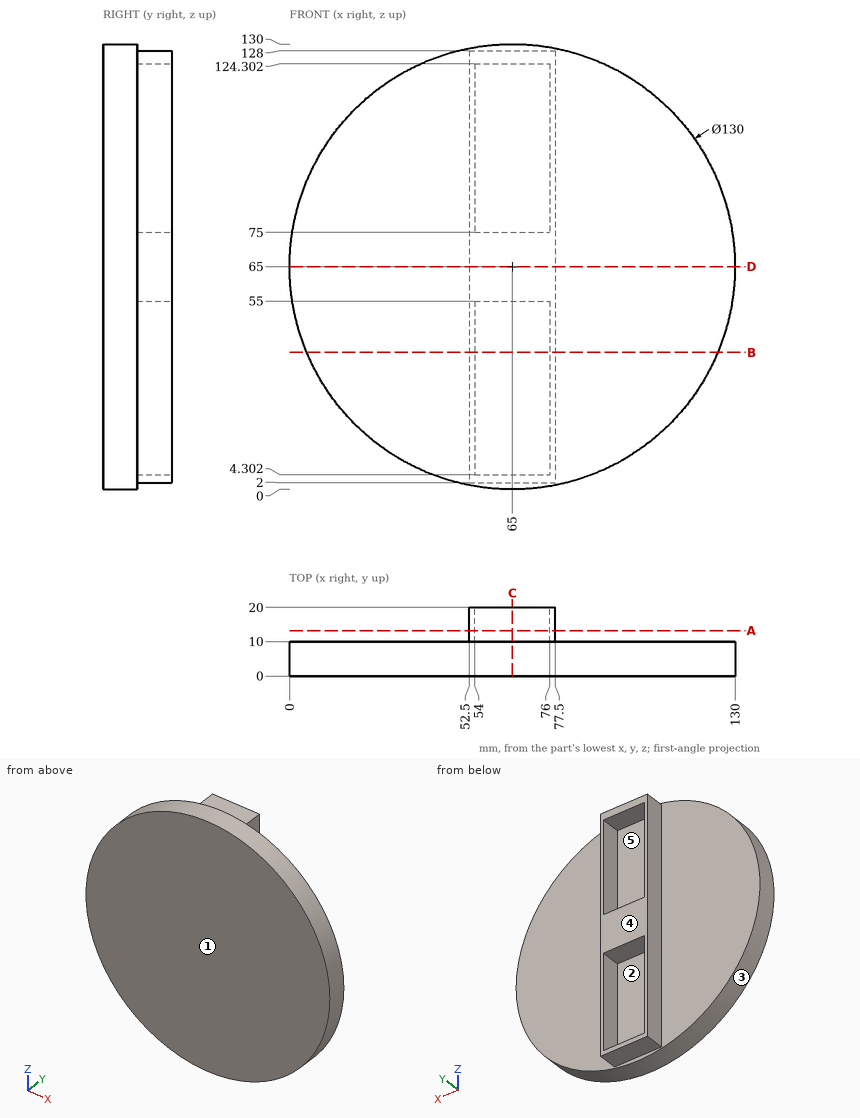
Check sheet for the drawn part. Datum: minimum x, y, z corner. Units: mm. A direction names the side the tool comes from. Round coordinates to 2 decimals unless told otherwise and drop trailing zeros. Write each loop counter-clockwise with the first axis right and the second up, starting at its lowest first coordinate (ties: lowest second). Pieces come first, ordered by that corner, then holes. Notation, with made-up numbers: (59.25, 70.5) - (69.25, 70.5) arc R12 ccw to (69.25, 91.5) - close; hole circle Ø9 at (-11.5, 62). An arc over 180 degrees is marked (long way). Write each question's results on one line, items separated by ' | '.
(1) Set-up check for the marked faces 4 and 5: record each of +Z, -Z, +X, -X, +Y, -Y from which the full face is reachable in a straight line by a thin tool's end or side.
Computed:
face 4: +Z, -Z, +X, -X, +Y | face 5: +Y
(2) Draft check along Z on the marked faces 1, 2 and 3. Enter one of: pulls with the +Z half, pulls with the -Z half, needs draft (parallel to the pull), parting line crosses it, or undercut.
Computed:
face 1: needs draft | face 2: undercut | face 3: parting line crosses it
(3) Sectioned sample at B-B, the plane z = 40. Enter the section's corners in (x, y).
Computed:
outline: (5, 0) - (125, 0) - (125, 10) - (77.5, 10) - (77.5, 20) - (76, 20) - (76, 10) - (54, 10) - (54, 20) - (52.5, 20) - (52.5, 10) - (5, 10) - close
(4) Thickness scan on probe 1 along Z at (x, y) = (65.5, 13.5); probe 2 along X at (y, z) = (12.5, 122); probe 3 along Y at (x, z) = (11, 91.5). Record the ranges inside material, lowest first. Write a range as from..to.
Computed:
probe 1: z = 2..4.3, 55..75, 124.3..128 | probe 2: x = 52.5..54, 76..77.5 | probe 3: y = 0..10
(5) Depth check by flat-ended pin: pin 1 Ø3 at (x, y) = (60.5, 16.5) entering from +Z; pin 2 Ø5 at (x, y) = (76.5, 9) entering from +Z; pin 3 Ø3 at (x, y) = (64.5, 13.5) entering from -Z; pin 4 Ø1.5 at (x, y) = (29.5, 12) entering from -Z. Enter the tip coordinate at first touch or a pass-through.
Computed:
pin 1: stops at z = 128 | pin 2: stops at z = 129.37 | pin 3: stops at z = 2 | pin 4: passes through
(6) Sectioned sample at C-C, the plane x = 65. Enter the section's corners in (y, z).
Computed:
outline: (0, 0) - (10, 0) - (10, 2) - (20, 2) - (20, 4.3) - (10, 4.3) - (10, 55) - (20, 55) - (20, 75) - (10, 75) - (10, 124.3) - (20, 124.3) - (20, 128) - (10, 128) - (10, 130) - (0, 130) - close
(7) Sectioned sample at A-A, the plane y = 13.25. Enter the section's corners in (x, z).
Computed:
outline: (52.5, 2) - (77.5, 2) - (77.5, 128) - (52.5, 128) - close; hole (54, 4.3) - (76, 4.3) - (76, 55) - (54, 55) - close; hole (54, 75) - (76, 75) - (76, 124.3) - (54, 124.3) - close
(8) Sectioned sample at D-D, the plane z = 65. Enter the section's corners in (x, y), plus the area to 3 significant figures.
Computed:
outline: (0, 0) - (130, 0) - (130, 10) - (77.5, 10) - (77.5, 20) - (52.5, 20) - (52.5, 10) - (0, 10) - close | area: 1,550 mm^2
